```python
from build123d import *

# Parameters (mm, degrees)
F0_W     = 548
F0_H     = 256
F0_R     = 3.25
F0_R_2   = 5.5
F1_DEPTH = 2
F2_SIZE  = 0.5


with BuildPart() as f1:
    # F0 (on Front) → F1 (new body)
    with BuildSketch(Plane.XZ):
        Rectangle(F0_W, F0_H)
        with Locations((-264, -119)):
            Circle(F0_R, mode=Mode.SUBTRACT)
        with Locations((-104, -119)):
            Circle(F0_R, mode=Mode.SUBTRACT)
        with Locations((56, -119)):
            Circle(F0_R, mode=Mode.SUBTRACT)
        with Locations((216, -119)):
            Circle(F0_R_2, mode=Mode.SUBTRACT)
        with Locations((266, -103)):
            Circle(F0_R, mode=Mode.SUBTRACT)
        with Locations((-264, 119)):
            Circle(F0_R, mode=Mode.SUBTRACT)
        with Locations((-104, 119)):
            Circle(F0_R, mode=Mode.SUBTRACT)
        with Locations((266, 0)):
            Circle(F0_R, mode=Mode.SUBTRACT)
        with Locations((56, 119)):
            Circle(F0_R, mode=Mode.SUBTRACT)
        with Locations((266, 103)):
            Circle(F0_R, mode=Mode.SUBTRACT)
        with Locations((216, 119)):
            Circle(F0_R_2, mode=Mode.SUBTRACT)
    extrude(amount=F1_DEPTH)

    # F2
    f2_edges = [f1.edges().sort_by_distance(p)[0] for p in [
        (-260.75, -1, 119),
        (-267.25, 0, 119),
        (-267.25, -2, 119),
        (-100.75, -1, 119),
        (-107.25, 0, 119),
        (-107.25, -2, 119),
        (59.25, -1, 119),
        (52.75, 0, 119),
        (52.75, -2, 119),
        (269.25, -1, 103),
        (262.75, 0, 103),
        (262.75, -2, 103),
        (269.25, -1, 0),
        (262.75, 0, 0),
        (262.75, -2, 0),
        (269.25, -1, -103),
        (262.75, 0, -103),
        (262.75, -2, -103),
        (59.25, -1, -119),
        (52.75, 0, -119),
        (52.75, -2, -119),
        (-100.75, -1, -119),
        (-107.25, 0, -119),
        (-107.25, -2, -119),
        (-260.75, -1, -119),
        (-267.25, 0, -119),
        (-267.25, -2, -119),
        (221.5, -1, 119),
        (210.5, 0, 119),
        (210.5, -2, 119),
        (221.5, -1, -119),
        (210.5, 0, -119),
        (210.5, -2, -119),
    ]]
    chamfer(f2_edges, length=F2_SIZE)


solid = f1.part
```
Part model, mm, in its own coordinate system. Give positions to 0.01 mm unless a question says otherwise; leave off trailing zeros. Loops run counter-clockwise (first coordinate to the right, second up) from the corner with the lowest first, then second, coordinate; pieces in that order, holes last. Notation, with made-up numbers: M 49.25,77 L 63.25,77 A16 ccw 63.25,102 Z; hole C 47.5,73.5 d3. An arc over 180 degrees is marked long. Return JSON: item names as keys, results as strings.
1) Saw through at A-A, the plane x = 216. List the corners of the cut face in (y, z).
Calculated:
{"outline": "M -2,-128 L 0,-128 L 0,-125 L -0.5,-124.5 L -1.5,-124.5 L -2,-125 Z; M -2,-113 L -1.5,-113.5 L -0.5,-113.5 L 0,-113 L 0,113 L -0.5,113.5 L -1.5,113.5 L -2,113 Z; M -2,125 L -1.5,124.5 L -0.5,124.5 L 0,125 L 0,128 L -2,128 Z"}
2) Pull direction Z, two halves, no side cores. Call faces 1 (the face through (-4, 0, 2)), 2 (the face through (215.284, -0.993, -113.547)): released by +Z, released by -Z, zero draft, split by the parting line, or undercut.
Calculated:
{"face 1": "zero draft", "face 2": "undercut"}
3) Drill centre lines: line 1 (Z direction, x = -264, y = -1.1); line 2 (Z direction, x = 266, y = -0.95); line 3 (Z direction, x = 216, y = -1.1). Where is each one in solid material? Low to high.
Calculated:
{"line 1": "z = -128 to -122.25, -115.75 to 115.75, 122.25 to 128", "line 2": "z = -128 to -106.25, -99.75 to -3.25, 3.25 to 99.75, 106.25 to 128", "line 3": "z = -128 to -124.5, -113.5 to 113.5, 124.5 to 128"}
